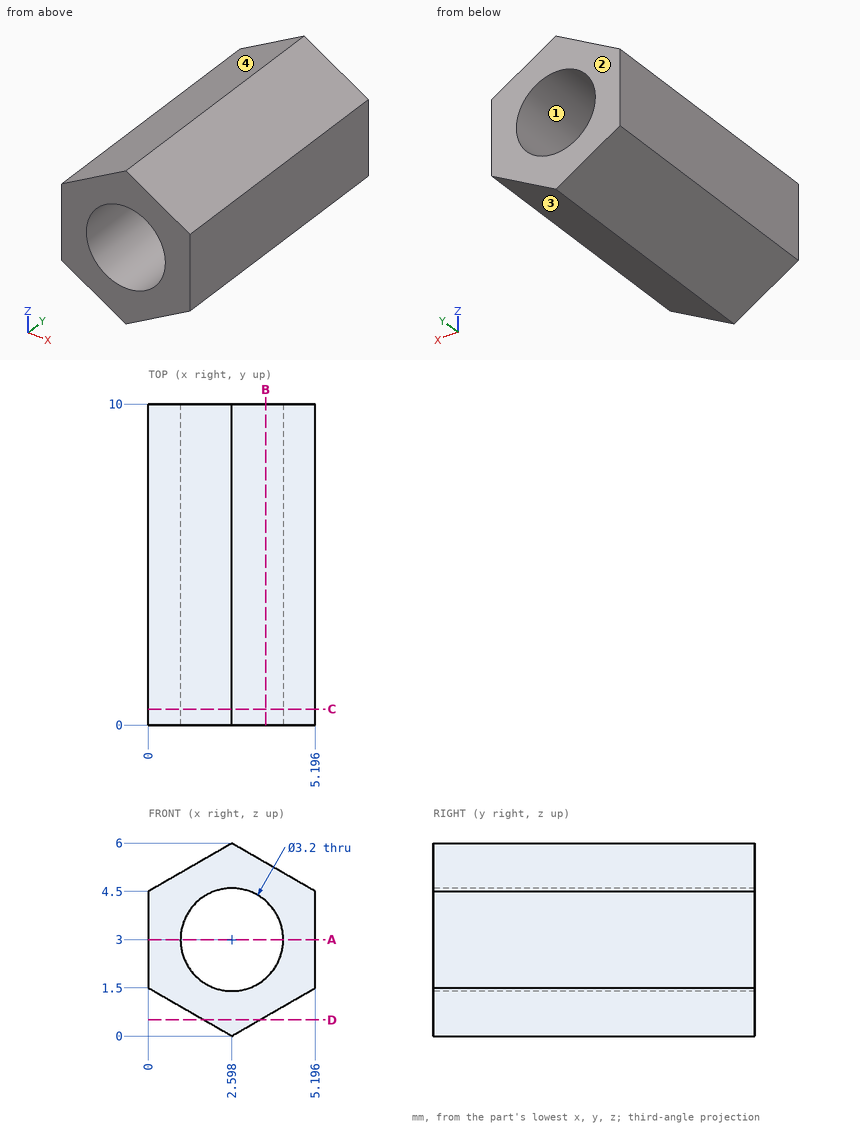
The drawing under review shows one solid part. Ordinate dimensions are in mm from its lowest x, y, z. Round coordinates to 2 decimals unless told otherwise and drop trailing zeros. Loops run counter-clockwise (first coordinate to the right, second up) from the corner with the lowest first, then second, coordinate; pieces in that order, holes last.
Item 1: Take a section at A-A (z = 3). Write out the cut boundary in (x, y).
Determined:
outline: (0, 0) - (1, 0) - (1, 10) - (0, 10) - close; (4.2, 0) - (5.2, 0) - (5.2, 10) - (4.2, 10) - close
Item 2: Take a section at C-C (y = 0.5). Write out the cut boundary in (x, z).
Determined:
outline: (0, 1.5) - (2.6, 0) - (5.2, 1.5) - (5.2, 4.5) - (2.6, 6) - (0, 4.5) - close; hole circle Ø3.2 at (2.6, 3)
Item 3: Mouldability with a two-part tool opening along Z and no side actions: class the marked faces 1, 2, 3 and 4 as released by +Z, released by -Z, zero draft, split by the parting line, or undercut.
Determined:
face 1: undercut
face 2: zero draft
face 3: released by -Z
face 4: released by +Z
Item 4: For line 1 (X direction, y = 5.75, z = 3); line 2 (X direction, y = 3.5, z = 3.9) (1 decimal); line 3 (Z direction, x = 3.45, y = 0.75) (1 decimal), list the stretches that pass through material, from the lowest coordinate up.
Determined:
line 1: x = 0 to 1, 4.2 to 5.2
line 2: x = 0 to 1.3, 3.9 to 5.2
line 3: z = 0.5 to 1.6, 4.4 to 5.5
Item 5: Take a section at B-B (x = 3.65). Write out the cut boundary in (y, z).
Determined:
outline: (0, 0.61) - (10, 0.61) - (10, 1.79) - (0, 1.79) - close; (0, 4.21) - (10, 4.21) - (10, 5.39) - (0, 5.39) - close
Item 6: Take a section at D-D (z = 0.5). Write out the cut boundary in (x, y).
Determined:
outline: (1.73, 0) - (3.46, 0) - (3.46, 10) - (1.73, 10) - close
